Answer from the drawing. Dimensions are ordinates in mm from the lowest x, y and z of the part. A direction names the side the tool comes from. Coordinates: 2 decimals unless noted, no trailing zeros. Order: outer loops, then holes, each group sorted by start corner. A loop starts at its lowest first (then second) coordinate and runs counter-clockwise, first axis right, second up. Notation, with made-up numbers: (-39, 83) - (-6, 83) arc R34 cw to (-6, 121) - close; hole circle Ø10 at (-35, -31.75). An arc over 180 degrees is marked (long way). Use a Markdown table: item, result. Add a question column.
Item 1: The part is cut by section A-A, the plane y = 8.45. Give the vertices of the cut face in (x, z).
Item 2: A flat-ended cylindrical pin translates along its axis: P1, Ø1.5, axis at x = 36.5, z = 2, coming from the -Y side. Find the tip coordinate at first contact, or state that the pin passes through.
Item 3: The part is cut by section C-C, the plane z = 2.85. Give the vertices of the cut face in (x, y).
Item 4: For the marked faces 5 and 6, determine the directions among +Z, -Z, +X, -X, +Y, -Y from which every point of the face is accessible in a straight line to the end or side of a thin tool.
Item 5: Find the intervals of material crossed by line 1 along X through (y, z) = (12.5, 3.5); line 2 along X through (y, z) = (6.5, 2.1) (1 decimal); line 3 along X through (y, z) = (9.25, 2), in increasing order.
Item 6: The part is cut by section D-D, the plane x = 28. Give the vertices of the cut face in (y, z), then the cut area to 3 significant figures.
Item 7: The mould has two halves that part along X. Classify the marked faces 1, 2, 3 and 4: released by +X, released by -X, zero draft, split by the parting line, or undercut.
Item 8: The part is cut by section B-B, the plane y = 4.25. Give the vertices of the cut face in (x, z).
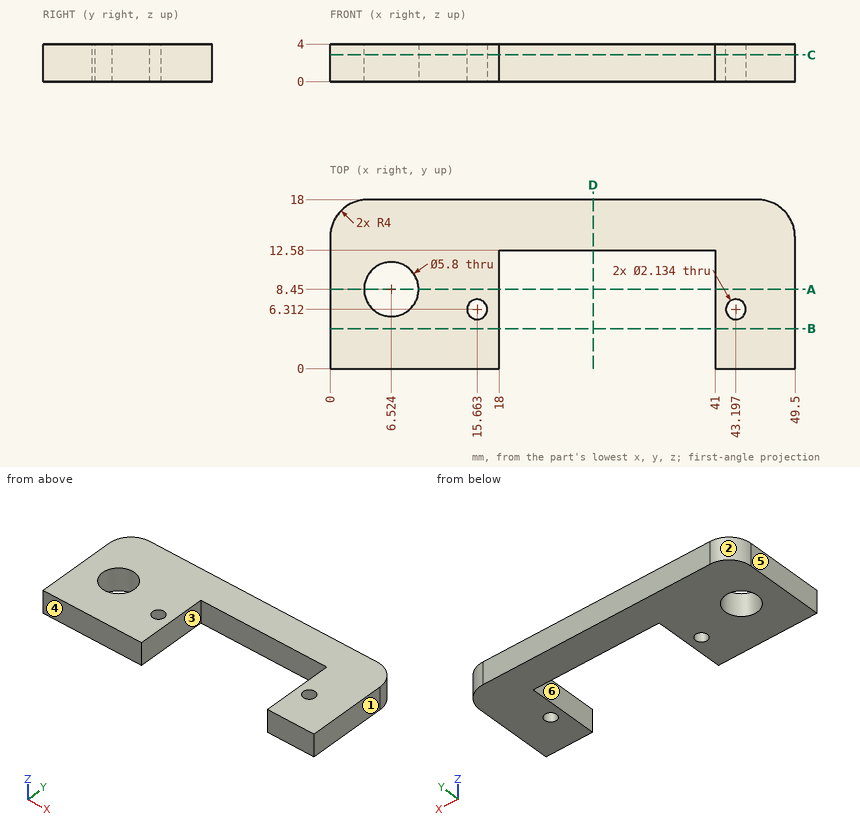
Solution:
| question | item | result |
|---|---|---|
| 1 | outline | (0, 0) - (3.62, 0) - (3.62, 4) - (0, 4) - close; (9.42, 0) - (18, 0) - (18, 4) - (9.42, 4) - close; (41, 0) - (49.5, 0) - (49.5, 4) - (41, 4) - close |
| 2 | P1 | stops at y = 12.58 |
| 3 | outline | (0, 0) - (18, 0) - (18, 12.58) - (41, 12.58) - (41, 0) - (49.5, 0) - (49.5, 14) arc R4 ccw to (45.5, 18) - (4, 18) arc R4 ccw to (0, 14) - close; hole circle Ø5.8 at (6.52, 8.45); hole circle Ø2.13 at (15.66, 6.31); hole circle Ø2.13 at (43.2, 6.31) |
| 4 | face 5 | +Z, -Z, -X, +Y, -Y |
| 4 | face 6 | +Z, -Z, -Y |
| 5 | line 1 | x = 0 to 18, 41 to 49.5 |
| 5 | line 2 | x = 0 to 4.4, 8.7 to 14.6, 16.7 to 18, 41 to 42.1, 44.2 to 49.5 |
| 5 | line 3 | x = 0 to 3.74, 9.31 to 18, 41 to 49.5 |
| 6 | outline | (12.58, 0) - (18, 0) - (18, 4) - (12.58, 4) - close |
| 6 | area | 21.7 mm2 |
| 7 | face 1 | released by +X |
| 7 | face 2 | released by -X |
| 7 | face 3 | undercut |
| 7 | face 4 | zero draft |
| 8 | outline | (0, 0) - (18, 0) - (18, 4) - (0, 4) - close; (41, 0) - (49.5, 0) - (49.5, 4) - (41, 4) - close |
